from build123d import *

# Parameters (mm, degrees)
F0_R     = 3.175
F1_DEPTH = 1.778
F2_R     = 2.3749
F3_DEPTH = 22.86
F4_R     = 2.286
F5_DEPTH = 3.175
F6_R     = 1.0922
F7_DEPTH = 27.814
F8_SIZE  = 0.635


with BuildPart() as f1:
    # F0 (on Front) → F1 (new body)
    with BuildSketch(Plane.XZ):
        Circle(F0_R)
    extrude(amount=F1_DEPTH)

    # F2 (on face) → F3 (join)
    with BuildSketch(Plane.XZ.offset(1.778)):
        Circle(F2_R)
    extrude(amount=F3_DEPTH)

    # F4 (on face) → F5 (join)
    with BuildSketch(Plane(origin=(0, 0, 0), x_dir=(-1, 0, 0), z_dir=(0, 1, 0))):
        Circle(F4_R)
    extrude(amount=F5_DEPTH)

    # F6 (on face) → F7 (cut, through all)
    with BuildSketch(Plane.XZ.offset(24.638)):
        Circle(F6_R)
    extrude(amount=-F7_DEPTH, mode=Mode.SUBTRACT)

    # F8
    f8_edges = [f1.edges().sort_by_distance(p)[0] for p in [
        (-2.3749, -24.638, 0),
    ]]
    chamfer(f8_edges, length=F8_SIZE)


solid = f1.part
Source: CAD feature listing. Evaluate the final solid. Frame: model axes, mm. A direction names the side the tool comes from. Round coordinates to 2 decimals unless told otherwise and drop trailing zeros. Loops run counter-clockwise (first coordinate to the right, second up) from the corner with the lowest first, then second, coordinate; pieces in that order, holes last. Notation, with made-up numbers: (25, 67.5) - (31, 67.5) arc R21 cw to (31, 79.5) - close; hole circle Ø6 at (8.25, 85). An arc over 180 degrees is marked (long way). Write item = value, one per line. Start each with the question number.
Item 1: Section query D-D on y = -20.5. Output: boundary loops of the cut face in (x, z).
Item 2: Mould query, pull axis X, two halves, no side actions, for faces 3 (the face through (1.04, -10.93, 0.33)), 4 (the face through (-1.75, -12.735, 1.605)), 5 (the face through (1.4, 0, -2.1)). Classes: released by +X, released by -X, zero draft, split by the parting line, or undercut.
Item 3: Section query C-C on y = 0.25. Output: boundary loops of the cut face in (x, z), plus the area to 3 significant figures.
Item 4: First-contact query: pin 1 Ø1 at (y, z) = (-21.5, -2.5) entering from -X; pin 2 Ø2 at (y, z) = (-20, -2.5) entering from -X; pin 3 Ø3 at (x, z) = (0.5, 0) entering from +Y (3 decimals); pin 4 Ø1 at (x, y) = (1.5, -1.5) entering from -Z. Flat tips, straight axial feed; report the tip coordinate or a pass-through.
Item 5: Reachability of faces 1 (the face through (0.5, 1.57, -2.23)), 2 (the face through (-0.69, -0.88, -3.1)) from +Z, -Z, +X, -X, +Y, -Y: full face, straight path, thin tool, end or side. Return the list, or none.
Item 6: Section query A-A on x = 0. Output: boundary loops of the cut face in (y, z) (3 decimals), plus the area to 3 significant figures.
Item 7: Section query B-B on z = 0. Output: boundary loops of the cut face in (x, y) (3 decimals).
Item 8: Material intervals for line 1 (Z direction, x = 0, y = -15); line 2 (Y direction, x = 1.5, z = 2.5); line 3 (Z direction, x = -0.75, y = -8.25), sorted ascending.
Results list:
q1.outline = circle Ø4.75 at (0, 0); hole circle Ø2.18 at (0, 0)
q2.face_3 = undercut
q2.face_4 = split by the parting line
q2.face_5 = zero draft
q3.outline = circle Ø4.57 at (0, 0); hole circle Ø2.18 at (0, 0)
q3.area = 12.7 mm²
q4.pin_1 = -1.28
q4.pin_2 = -1.84
q4.pin_3 = 3.175
q4.pin_4 = -3.01
q5.face_1 = +Y
q5.face_2 = +Y, -Y
q6.outline = (-24.638, -1.74) - (-24.003, -2.375) - (-1.778, -2.375) - (-1.778, -3.175) - (0, -3.175) - (0, -2.286) - (3.175, -2.286) - (3.175, -1.092) - (-24.638, -1.092) - close; (-24.638, 1.092) - (3.175, 1.092) - (3.175, 2.286) - (0, 2.286) - (0, 3.175) - (-1.778, 3.175) - (-1.778, 2.375) - (-24.003, 2.375) - (-24.638, 1.74) - close
q6.area = 73.2 mm²
q7.outline = (-3.175, -1.778) - (-2.375, -1.778) - (-2.375, -24.003) - (-1.74, -24.638) - (-1.092, -24.638) - (-1.092, 3.175) - (-2.286, 3.175) - (-2.286, 0) - (-3.175, 0) - close; (1.092, -24.638) - (1.74, -24.638) - (2.375, -24.003) - (2.375, -1.778) - (3.175, -1.778) - (3.175, 0) - (2.286, 0) - (2.286, 3.175) - (1.092, 3.175) - close
q8.line_1 = -2.37 to -1.09, 1.09 to 2.37
q8.line_2 = -1.78 to 0
q8.line_3 = -2.25 to -0.79, 0.79 to 2.25
